```python
from build123d import *

# Parameters (mm, degrees)
BOSS_EXTRUDE1_DEPTH = 10
BOSS_EXTRUDE2_DEPTH = 10
SKETCH3_W           = 10
SKETCH3_H           = 10
REVOLVE1_ANGLE      = 10
SKETCH4_W           = 10
SKETCH4_H           = 10
CUT_REVOLVE1_ANGLE  = 12
SKETCH5_W           = 10
SKETCH5_H           = 10
REVOLVE2_ANGLE      = 90
FILLET1_R           = 2.5


with BuildPart() as part:
    # Sketch1 → Boss-Extrude1 (new body)
    with BuildSketch(Plane(origin=(0, 0, 0), x_dir=(1, 0, 0), z_dir=(0, 1, 0))):
        with BuildLine():
            ThreePointArc((10, 104.522724802), (44.760729067, 94.981456787), (74.246212025, 74.246212025))
            Line((74.246212025, 74.246212025), (88.388347648, 88.388347648))
            ThreePointArc((88.388347648, 88.388347648), (0, 125), (-88.388347648, 88.388347648))
            Line((-88.388347648, 88.388347648), (-74.246212025, 74.246212025))
            ThreePointArc((-74.246212025, 74.246212025), (-44.760729067, 94.981456787), (-10, 104.522724802))
            Line((-10, 104.522724802), (-10, 105))
            Line((-10, 105), (7e-08, 105))
            Line((7e-08, 105), (10, 105))
            Line((10, 105), (10, 104.522724802))
        make_face()
        with BuildLine():
            ThreePointArc((-10, 99.498743711), (0, 100), (10, 99.498743711))
            Line((10, 99.498743711), (10, 104.522724802))
            ThreePointArc((10, 104.522724802), (5.005691586, 104.880613327), (7e-08, 105))
            ThreePointArc((7e-08, 105), (-5.005691516, 104.88061333), (-10, 104.522724802))
            Line((-10, 104.522724802), (-10, 99.498743711))
        make_face()
        with BuildLine():
            ThreePointArc((7e-08, 105), (5.005691586, 104.880613327), (10, 104.522724802))
            Line((10, 104.522724802), (10, 105))
            Line((10, 105), (7e-08, 105))
        make_face()
        with BuildLine():
            Line((-10, 105), (-10, 104.522724802))
            ThreePointArc((-10, 104.522724802), (-5.005691516, 104.88061333), (7e-08, 105))
            Line((7e-08, 105), (-10, 105))
        make_face()
    extrude(amount=BOSS_EXTRUDE1_DEPTH)

    # Sketch2 → Boss-Extrude2 (add)
    with BuildSketch(Plane(origin=(0, 10, 0), x_dir=(1, 0, 0), z_dir=(0, 1, 0))):
        with BuildLine():
            Line((-88.388347648, 88.388347648), (-74.246212025, 74.246212025))
            ThreePointArc((-74.246212025, 74.246212025), (-44.760729067, 94.981456787), (-10, 104.522724802))
            Line((-10, 104.522724802), (-10, 99.498743711))
            ThreePointArc((-10, 99.498743711), (0, 100), (10, 99.498743711))
            Line((10, 99.498743711), (10, 104.522724802))
            ThreePointArc((10, 104.522724802), (44.760729067, 94.981456787), (74.246212025, 74.246212025))
            Line((74.246212025, 74.246212025), (88.388347648, 88.388347648))
            ThreePointArc((88.388347648, 88.388347648), (0, 125), (-88.388347648, 88.388347648))
        make_face()
        with BuildLine():
            ThreePointArc((-10, 104.522724802), (-44.760729067, 94.981456787), (-74.246212025, 74.246212025))
            Line((-74.246212025, 74.246212025), (-70.710678119, 70.710678119))
            ThreePointArc((-70.710678119, 70.710678119), (-42.845554854, 90.356286053), (-10, 99.498743711))
            Line((-10, 99.498743711), (-10, 104.522724802))
        make_face()
        with BuildLine():
            Line((70.710678119, 70.710678119), (74.246212025, 74.246212025))
            ThreePointArc((74.246212025, 74.246212025), (44.760729067, 94.981456787), (10, 104.522724802))
            Line((10, 104.522724802), (10, 99.498743711))
            ThreePointArc((10, 99.498743711), (42.845554854, 90.356286053), (70.710678119, 70.710678119))
        make_face()
    extrude(amount=BOSS_EXTRUDE2_DEPTH)

    # Sketch3 → Revolve1 (revolve)
    with BuildSketch(Plane(origin=(0, 0, 0), x_dir=(0.7071067811865512, 0, 0.7071067811865438), z_dir=(-0.7071067811865438, 0, 0.7071067811865512))):
        Polygon((-120, 17.5), (-120, 12.5), (-110, 12.5), (-105, 12.5), (-105, 17.5), align=None)
        with Locations((-115, 7.5)):
            Rectangle(SKETCH3_W, SKETCH3_H)
    revolve(axis=Axis((0, 0, 0), (0, 1, 0)), revolution_arc=REVOLVE1_ANGLE)

    # Sketch4 → Cut-Revolve1 (revolve, cut)
    with BuildSketch(Plane(origin=(0, 0, 0), x_dir=(0.7071067811865507, 0, -0.7071067811865445), z_dir=(0.7071067811865445, 0, 0.7071067811865507))):
        Polygon((105, 12.5), (110, 12.5), (120, 12.5), (120, 17.5), (105, 17.5), align=None)
        with Locations((115, 7.5)):
            Rectangle(SKETCH4_W, SKETCH4_H)
    revolve(axis=Axis((0, 0, 0), (0, 1, 0)), revolution_arc=CUT_REVOLVE1_ANGLE, mode=Mode.SUBTRACT)

    # Sketch5 → Revolve2 (revolve)
    with BuildSketch(Plane(origin=(0, 0, 0), x_dir=(0.7071067811865512, 0, 0.7071067811865438), z_dir=(-0.7071067811865438, 0, 0.7071067811865512))):
        with Locations((-125, 10)):
            Rectangle(SKETCH5_W, SKETCH5_H)
    revolve(axis=Axis((0, 0, 0), (0, -1, 0)), revolution_arc=REVOLVE2_ANGLE)

    # Fillet1
    fillet1_edges = [part.edges().sort_by_distance(p)[0] for p in [
        (-42.845554854, 10, -90.356286053),
        (42.845554854, 10, -90.356286053),
    ]]
    fillet(fillet1_edges, radius=FILLET1_R)


solid = part.part
```
Geometry: final body of the model. Coordinates: model frame, mm. A direction names the side the tool comes from. Round coordinates to 2 decimals unless told otherwise and drop trailing zeros. Write each loop counter-clockwise with the first axis right and the second up, starting at its lowest first coordinate (ties: lowest second). Pieces come first, ordered by that corner, then holes. Notation, with made-up numbers: (-38.75, 85) -> (-2.75, 85) arc R18 cw to (-2.75, 106) -> close; hole circle Ø6 at (-19, 49.25). An arc over 180 degrees is marked (long way). Return JSON: item names as keys, results as strings.
Q1. Mould query, pull axis X, two halves, no side actions, for faces 4 (the flat face through (77, 10, -77)), 5 (the flat face through (72, 2.5, -89)), 6 (the flat face through (0, 5, -126)). Classes: +X half, -X half, draft (parallel to the pull), parting line (faces both ways), or undercut.
From the geometry:
{"face 4": "+X half", "face 5": "undercut", "face 6": "draft"}
Q2. Section A-A on x = 1.5. Return the cut outline in (y, z).
From the geometry:
{"outline": "(0, -124.99) -> (5, -124.99) -> (5, -129.99) -> (15, -129.99) -> (15, -124.99) -> (20, -124.99) -> (20, -99.99) -> (0, -99.99) -> close"}
Q3. First-contact query: pin 1 Ø2.5 at (y, z) = (3, -101.5) entering from +X; pin 2 Ø8 at (y, z) = (2.5, -109.5) entering from -X (3 decimals); pin 3 Ø6 at (x, z) = (-86, -71.5) entering from -Y. Flat tips, straight axial feed; report the tip coordinate or a pass-through.
From the geometry:
{"pin 1": "x = 74.67", "pin 2": "x = -74.725", "pin 3": "y = 2.5"}
Q4. Section B-B on z = -66. Return the cut outline in (x, y).
From the geometry:
{"outline": "(-94.26, 2.5) -> (-88, 2.5) -> (-88, 12.5) -> (-81.66, 12.5) -> (-81.66, 17.5) -> (-94.26, 17.5) -> close"}
Q5. Set-up query: faces 1 (the cylindrical face through (-80.352, 15.035, -67.591)), 2 (the flat face through (10, 5, -102)), 3 (the cylindrical face through (69.35, 7.57, -85.384)). Return all of +Z, -Z, +X, -X, +Y, -Y with unobstructed straight access to the full face (end or side cutting, diameter ignored); none if empty.
From the geometry:
{"face 1": "+Z, +Y, -Y", "face 2": "+Z, -Y", "face 3": "none"}
Q6. Ray query, line 1 (X direction, y = 11, z = -76.5); line 2 (X direction, y = 15.5, z = -85); line 3 (Y direction, x = 47.5, z = -92). Return the intervals inside material, ascending.
From the geometry:
{"line 1": "-92.45 to -79.04, -76.5 to -65.18, 65.18 to 76.5", "line 2": "-85 to -52.68, 52.68 to 61.64, 84.71 to 85", "line 3": "10 to 20"}
